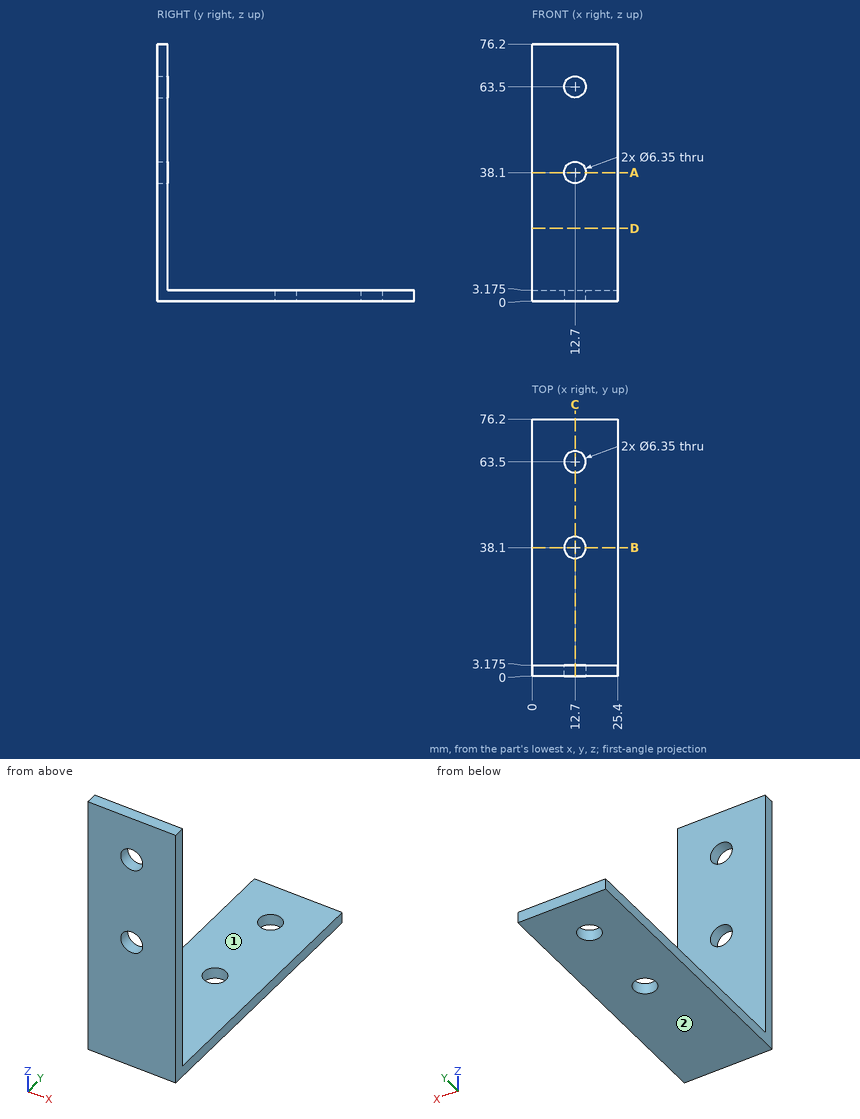
Design review of the part shown in the three views and the two pictorial views. Dimensions are in mm from the part's minimum x, y and z. A direction names the side the tool comes from. Round coordinates to 2 decimals unless told otherwise and drop trailing zeros. Order: outer loops, then holes, each group sorted by start corner. A loop starts at its lowest first (then second) coordinate and runs counter-clockwise, first axis right, second up.
Q1. Wall thickness on line 1 (Y direction, x = 12.7, z = 1.7) (3 decimals); line 2 (Z direction, x = 17.25, y = 54) (3 decimals): over which ranges is each line inside the solid? List them lowest first.
Findings below:
line 1: y = 0 to 34.925, 41.275 to 60.325, 66.675 to 76.2
line 2: z = 0 to 3.175
Q2. We need section D-D, the plane z = 21.5. Give the boundary of the cut face in (x, y) (3 decimals), plus the area to 3 significant figures.
Findings below:
outline: (0, 0) - (25.4, 0) - (25.4, 3.175) - (0, 3.175) - close
area: 80.6 mm2
Q3. We need section C-C, the plane x = 12.7. Give the boundary of the cut face in (y, z) (3 decimals).
Findings below:
outline: (0, 0) - (34.925, 0) - (34.925, 3.175) - (3.175, 3.175) - (3.175, 34.925) - (0, 34.925) - close; (0, 41.275) - (3.175, 41.275) - (3.175, 60.325) - (0, 60.325) - close; (0, 66.675) - (3.175, 66.675) - (3.175, 76.2) - (0, 76.2) - close; (41.275, 0) - (60.325, 0) - (60.325, 3.175) - (41.275, 3.175) - close; (66.675, 0) - (76.2, 0) - (76.2, 3.175) - (66.675, 3.175) - close
Q4. We need section A-A, the plane z = 38.1. Give the boundary of the cut face in (x, y) (3 decimals), plus the area to 3 significant figures.
Findings below:
outline: (0, 0) - (9.525, 0) - (9.525, 3.175) - (0, 3.175) - close; (15.875, 0) - (25.4, 0) - (25.4, 3.175) - (15.875, 3.175) - close
area: 60.5 mm2
Q5. Insertion check: P1, Ø7.5, axis at x = 12.7, z = 38.1, coming from the +Y side (3 decimals); P2, Ø2, axis at x = 10.5, y = 61.5, coming from the +Z side (3 decimals). Each pin has a flat end and moves straight along its axis. Give the tip position at first contact, or say it passes through.
Findings below:
P1: stops at y = 3.175
P2: stops at z = 3.175
Q6. Machinability: for the marked faces 1 and 2, which of the approach directions +Z, -Z, +X, -X, +Y, -Y give a long, thin tool a straight path to every point of the face, cutting with its end or side? Answer none if there is none.
Findings below:
face 1: +Z, +X, -X, +Y
face 2: -Z, +X, -X, +Y, -Y
